Source: CAD feature listing. Evaluate the final solid. Frame: model axes, mm. Face numbers are marked on the shaded views. Give positions to 0.01 mm unless a question says otherwise; leave off trailing zeros. Order: outer loops, then holes, each group sorted by start corner. A loop starts at its lowest first (then second) coordinate and runs counter-clockwise, first axis right, second up.
1) Draft query along X for the marked faces 1, 2 and 3. Return one class per face: released by +X, released by -X, zero draft, split by the parting line, or undercut.
2) Section A-A, the plane x = 0. Return loops of the section in (y, z).
3) Section D-D, the plane y = 5.5. Return loops of the section in (x, z).
4) Material intervals for line 1 (Y direction, x = 0, z = 19); line 2 (Y direction, x = 0, z = 42); line 3 (Z direction, x = -6.75, y = -8), sorted ascending.
5) Section C-C, the plane z = 48. Return loops of the section in (x, y), plus the area to 3 significant figures.
6) First-contact query: P1, Ø10, axis at x = -5.5, z = 27, coming from the -Y side; P2, Ø4, axis at x = -0.5, z = 18.5, coming from the +Y side; P3, Ø4, axis at x = 3.5, y = 3.5, coming from the -Z side; P4, Ø8, axis at y = -3, z = 39.5, coming from the -X side. Flat tips, straight axial feed; report the tip coordinate or a pass-through.
```python
from build123d import *

# Parameters (mm, degrees)
F3_D     = 6.8
F3_DEPTH = 20
F3_TIP   = 2.0429261047
F5_D     = 8
F5_DEPTH = 35
F5_TIP   = 2.4034424761


with BuildPart() as f1:
    # F0 (on Front) → F1 (revolve)
    with BuildSketch(Plane.XZ):
        Polygon((0, 53), (0, 0), (6.5, 0), (6.5, 50), (12.5, 50), (12.5, 53), align=None)
    revolve(axis=Axis((0, 0, 35.806838423), (0, 0, 1)))

    # F3
    with Locations(Plane.XY.offset(53)):
        with Locations((0, 0)):
            Hole(F3_D / 2, depth=F3_DEPTH)
            with Locations((0, 0, -(F3_DEPTH + F3_TIP / 2))):  # 118° drill point
                Cone(0, F3_D / 2, F3_TIP, mode=Mode.SUBTRACT)

    # F5
    with Locations(Plane(origin=(0, 0, 0), x_dir=(1, 0, 0), z_dir=(0, 0, -1))):
        with Locations((0, 0)):
            Hole(F5_D / 2, depth=F5_DEPTH)
            with Locations((0, 0, -(F5_DEPTH + F5_TIP / 2))):  # 118° drill point
                Cone(0, F5_D / 2, F5_TIP, mode=Mode.SUBTRACT)


solid = f1.part
```
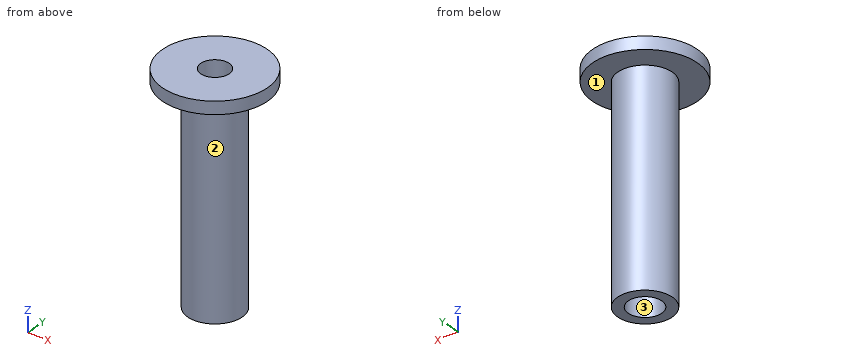
From the geometry:
1. face 1: zero draft
1. face 2: split by the parting line
1. face 3: undercut
2. outline: (-12.5, 50) - (-6.5, 50) - (-6.5, 0) - (-4, 0) - (-4, 35) - (-3.4, 35.36) - (-3.4, 53) - (-12.5, 53) - close; (3.4, 35.36) - (4, 35) - (4, 0) - (6.5, 0) - (6.5, 50) - (12.5, 50) - (12.5, 53) - (3.4, 53) - close
3. outline: (-11.22, 50) - (-3.46, 50) - (-3.46, 0) - (3.46, 0) - (3.46, 50) - (11.22, 50) - (11.22, 53) - (-11.22, 53) - close
4. line 1: y = -6.5 to -4, 4 to 6.5
4. line 2: y = -6.5 to -3.4, 3.4 to 6.5
4. line 3: z = 50 to 53
5. outline: circle Ø13 at (0, 0); hole circle Ø6.8 at (0, 0)
5. area: 96.4 mm2
6. P1: stops at y = -6.48
6. P2: stops at y = 6.5
6. P3: stops at z = 0
6. P4: stops at x = -6.5
